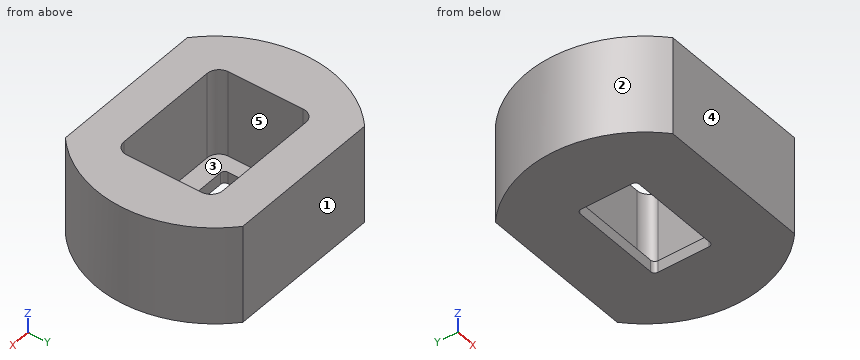
from build123d import *

# Parameters (mm, degrees)
F2_DEPTH = 25
F3_DEPTH = 22
F5_DEPTH = 3


with BuildPart() as f2:
    # F0 (on Top) → F2 (new body)
    with BuildSketch(Plane.XY):
        with BuildLine():
            Line((19.843135, 22.5), (-19.843135, 22.5))
            ThreePointArc((-19.843135, 22.5), (-30, 0), (-19.843135, -22.5))
            Line((-19.843135, -22.5), (19.843135, -22.5))
            ThreePointArc((19.843135, -22.5), (30, 0), (19.843135, 22.5))
        make_face()
    extrude(amount=-F2_DEPTH)

    # F1 (on face) → F3 (cut)
    with BuildSketch(Plane.XY):
        with BuildLine():
            ThreePointArc((-16.5, -9.5), (-15.62132, -11.62132), (-13.5, -12.5))
            Line((-13.5, -12.5), (13.5, -12.5))
            ThreePointArc((13.5, -12.5), (15.62132, -11.62132), (16.5, -9.5))
            Line((16.5, -9.5), (16.5, 9.5))
            ThreePointArc((16.5, 9.5), (15.62132, 11.62132), (13.5, 12.5))
            Line((13.5, 12.5), (-13.5, 12.5))
            ThreePointArc((-13.5, 12.5), (-15.62132, 11.62132), (-16.5, 9.5))
            Line((-16.5, 9.5), (-16.5, -9.5))
        make_face()
    extrude(amount=-F3_DEPTH, mode=Mode.SUBTRACT)

    # F4 (on face) → F5 (cut, through all)
    with BuildSketch(Plane(origin=(0, 0, -25), x_dir=(1, 0, 0), z_dir=(0, 0, -1))):
        with BuildLine():
            ThreePointArc((-12.5, -6.5), (-12.207107, -7.207107), (-11.5, -7.5))
            Line((-11.5, -7.5), (11.5, -7.5))
            ThreePointArc((11.5, -7.5), (12.207107, -7.207107), (12.5, -6.5))
            Line((12.5, -6.5), (12.5, 6.5))
            ThreePointArc((12.5, 6.5), (12.207107, 7.207107), (11.5, 7.5))
            Line((11.5, 7.5), (-11.5, 7.5))
            ThreePointArc((-11.5, 7.5), (-12.207107, 7.207107), (-12.5, 6.5))
            Line((-12.5, 6.5), (-12.5, -6.5))
        make_face()
    extrude(amount=-F5_DEPTH, mode=Mode.SUBTRACT)


solid = f2.part
The listing builds one solid part. Answer for the finished solid, in the listing's coordinates (mm). Face numbers are marked on the shaded views. A direction names the side the tool comes from. Give positions to 0.01 mm unless a question says otherwise; leave off trailing zeros. Write each loop counter-clockwise with the first axis right and the second up, starting at its lowest first coordinate (ties: lowest second). Pieces come first, ordered by that corner, then holes.
Item 1: Section B-B, the plane y = 0 is taken. Write down the section's boundary in (x, z).
Item 2: Section C-C, the plane z = -10 is taken. Write down the section's boundary in (x, y).
Item 3: Find the intervals of material crossed by line 1 along Y through (x, z) = (3, -11.25); line 2 along Z through (x, y) = (-11, 8); line 3 along X through (y, z) = (-11, -15), in increasing order.
Item 4: Which of the six approach directions +Z, -Z, +X, -X, +Y, -Y give full straight-line access (tool end or side, diameter ignored) to the marked faces 4 and 5?
Item 5: Determine the mould class of the marked faces 1, 2 and 3 for opening direction X: released by +X, released by -X, zero draft, split by the parting line, or undercut.
Item 6: Flat-ended cylindrical pins translate along their axes: P1, Ø7.5, axis at x = 2, y = 0.5, coming from the +Z side; P2, Ø3.5, axis at y = -1.5, z = -24, coming from the -X side; P3, Ø4, axis at y = -6, z = -19, coming from the -X side; P4, Ø1.5, axis at y = -10.5, z = -10.5, coming from the +X side. Find the tip coordinate at first contact, or state that the pin passes through.
Item 7: Section A-A, the plane x = 9 is taken. Write down the section's boundary in (y, z).
Item 8: Section D-D, the plane x = -21.5 is taken. Write down the section's boundary in (y, z), plus the area to 3 significant figures.
Completed:
1. outline: (-30, -25) - (-12.5, -25) - (-12.5, -22) - (-16.5, -22) - (-16.5, 0) - (-30, 0) - close; (12.5, -25) - (30, -25) - (30, 0) - (16.5, 0) - (16.5, -22) - (12.5, -22) - close
2. outline: (-19.84, -22.5) - (19.84, -22.5) arc R30 ccw to (19.84, 22.5) - (-19.84, 22.5) arc R30 ccw to start; hole (-16.5, -9.5) arc R3 ccw to (-13.5, -12.5) - (13.5, -12.5) arc R3 ccw to (16.5, -9.5) - (16.5, 9.5) arc R3 ccw to (13.5, 12.5) - (-13.5, 12.5) arc R3 ccw to (-16.5, 9.5) - close
3. line 1: y = -22.5 to -12.5, 12.5 to 22.5
3. line 2: z = -25 to -22
3. line 3: x = -27.91 to -16.1, 16.1 to 27.91
4. face 4: +Z, -Z, +X, -X, -Y
4. face 5: +Z
5. face 1: zero draft
5. face 2: released by -X
5. face 3: undercut
6. P1: passes through
6. P2: stops at x = -30
6. P3: stops at x = -29.73
6. P4: stops at x = 28.37
7. outline: (-22.5, -25) - (-7.5, -25) - (-7.5, -22) - (-12.5, -22) - (-12.5, 0) - (-22.5, 0) - close; (7.5, -25) - (22.5, -25) - (22.5, 0) - (12.5, 0) - (12.5, -22) - (7.5, -22) - close
8. outline: (-20.92, -25) - (20.92, -25) - (20.92, 0) - (-20.92, 0) - close
8. area: 1,050 mm2
